Check sheet for the modelled part. Datum: model origin and axes. Units: mm. A direction names the side the tool comes from. Give positions to 0.01 mm unless a question says otherwise; leave off trailing zeros. Write each loop counter-clockwise with the first axis right and the second up, starting at its lowest first coordinate (ties: lowest second). Pieces come first, ordered by that corner, then holes. Notation, with made-up numbers: (63, 54.25) -> (78, 54.25) arc R25 cw to (78, 74.25) -> close; hole circle Ø4 at (-29, -14). An arc over 180 degrees is marked (long way). Write each question's results on one line, items separated by ' | '. Start each with the question number.
Autodesk Inventor part; units mm, degrees
sketch "Sketch_2" plane through (0, 0, 0) normal (0, 1, 0) x (-1, 0, 0)
  line L0 (0.7786, 2.7778) -> (0.7786, 3.2051)
  line L1 (0.7786, 3.2051) -> (-0.5889, 3.2051)
  arc A0 (-0.5889, 3.2051) -> (-1.3581, 2.4359) centre (-0.5889, 2.4359) ccw
  line L2 (-1.3581, 2.4359) -> (-1.3581, 0.7692)
  arc A1 (-1.7, 0.4274) -> (-1.3581, 0.7692) centre (-1.7, 0.7692) ccw
  line L3 (-1.7, 0.4274) -> (-11.7, 0.4274)
  arc A2 (-12.0419, 0.7692) -> (-11.7, 0.4274) centre (-11.7, 0.7692) ccw
  line L4 (-12.0419, 0.7692) -> (-12.0419, 2.4359)
  arc A3 (-12.0419, 2.4359) -> (-12.8111, 3.2051) centre (-12.8111, 2.4359) ccw
  line L5 (-12.8111, 3.2051) -> (-14.1786, 3.2051)
  line L6 (-14.1786, 3.2051) -> (-14.1786, 2.7778)
  line L7 (-14.1786, 2.7778) -> (-12.8111, 2.7778)
  arc A4 (-12.4692, 2.4359) -> (-12.8111, 2.7778) centre (-12.8111, 2.4359) ccw
  line L8 (-12.4692, 2.4359) -> (-12.4692, 0.7692)
  arc A5 (-12.4692, 0.7692) -> (-11.7, 0) centre (-11.7, 0.7692) ccw
  line L9 (-11.7, 0) -> (-1.7, 0)
  arc A6 (-1.7, 0) -> (-0.9308, 0.7692) centre (-1.7, 0.7692) ccw
  line L10 (-0.9308, 0.7692) -> (-0.9308, 2.4359)
  arc A7 (-0.5889, 2.7778) -> (-0.9308, 2.4359) centre (-0.5889, 2.4359) ccw
  line L11 (-0.5889, 2.7778) -> (0.7786, 2.7778)
  dimension "d14" = 10
extrude "Extrusion1" add sketch "Sketch_2" along normal blind 159
sketch "Sketch_6" plane through (0, 0, 0) normal (0, 0, 1) x (1, 0, 0)
  arc A0 (4.05, 4.6232) -> (9.95, 4.6232) centre (7, 4.6232) ccw
  line L0 (9.95, 4.6232) -> (9.95, 19.1463)
  arc A1 (9.95, 19.1463) -> (4.05, 19.1463) centre (7, 19.1463) ccw
  line L1 (4.05, 19.1463) -> (4.05, 4.6232)
  dimension "d13" = 2.95
extrude "Extrusion2" cut sketch "Sketch_6" along normal blind 2
pattern_linear "Rectangular Pattern1" count 80 spacing 22.6 along (0, 1, 0) of "Extrusion2"
properties part number "PP0735H(1)" material "Ouro"
Item 1: Section check A-A on x = 7. Count the separate pieces of the cut face and the enclosed holes in it, then the cut area to 3 significant figures.
Item 2: Depth check by flat-ended pin: pin 1 Ø1.1 at (x, y) = (14, 79.5) entering from -Z; pin 2 Ø5 at (x, y) = (7.5, 39.5) entering from +Z; pin 3 Ø0.5 at (y, z) = (82, 0) entering from -X; pin 4 Ø4 at (x, y) = (11.5, 32.5) entering from -Z. Enter the tip coordinate at first touch or a pass-through.
Item 3: Set-up check for faces 3 (the flat face through (3, 78, 0)), 4 (the flat face through (3, 78, 0.427)), 5 (the cylindrical face through (7.065, 114.674, 0.211)): record each of +Z, -Z, +X, -X, +Y, -Y from which the full face is reachable in a straight line by a thin tool's end or side.
Item 4: Thickness scan on probe 1 along X at (y, z) = (127.5, 0.95); probe 2 along Z at (x, y) = (13.5, 137); probe 3 along Z at (x, y) = (8.5, 137). Record the ranges inside material, lowest first. Write a range as from..to.
Item 5: Mould release check, pull along X, two halves, no side actions. Record for faces 1 (the flat face through (6.7, 0, 0.2)), 2 (the cylindrical face through (7.065, 69.474, 0.211)): pulls with the +X half, pulls with the -X half, needs draft (parallel to the pull), parting line crosses it, or undercut.
Item 6: Section check B-B on y = 100. Record the boundary of the cut face in (x, z).
Check sheet entries:
1) separate pieces: 8 | enclosed holes: 0 | area: 6.85 mm^2
2) pin 1: stops at z = 2.78 | pin 2: stops at z = 0.43 | pin 3: stops at x = 1.13 | pin 4: stops at z = 0
3) face 3: -Z, +X, -X, +Y, -Y | face 4: +Z, +Y, -Y | face 5: +Z, -Z
4) probe 1: x = 0.93..1.36, 12.04..12.47 | probe 2: z = 2.78..3.21 | probe 3: z = 0..0.43
5) face 1: needs draft | face 2: undercut
6) outline: (-0.78, 2.78) -> (0.59, 2.78) arc R0.34 cw to (0.93, 2.44) -> (0.93, 0.77) arc R0.77 ccw to (1.7, 0) -> (4.05, 0) -> (4.05, 0.43) -> (1.7, 0.43) arc R0.34 cw to (1.36, 0.77) -> (1.36, 2.44) arc R0.77 ccw to (0.59, 3.21) -> (-0.78, 3.21) -> close; (9.95, 0) -> (11.7, 0) arc R0.77 ccw to (12.47, 0.77) -> (12.47, 2.44) arc R0.34 cw to (12.81, 2.78) -> (14.18, 2.78) -> (14.18, 3.21) -> (12.81, 3.21) arc R0.77 ccw to (12.04, 2.44) -> (12.04, 0.77) arc R0.34 cw to (11.7, 0.43) -> (9.95, 0.43) -> close
